Here's how the part is built. I have some questions about the finished solid (model axes, mm). Coordinates: 2 decimals unless noted, no trailing zeros. Answer in a Markdown table with one row per item. Add a question column.
Item 1: If I drill on probe 1 along Z at (x, y) = (-3, -392); probe 2 along X at (y, z) = (399, -3.5); probe 3 along X at (y, z) = (5.5, 25.5), over which ranges is the centre line in solid material (lowest first)? Write a range as from..to.
Item 2: Imagine slicing it at A-A (y = -155). State how many separate pieces and enclosed holes the cut face has, plus the area to 3 significant figures.
Item 3: I'm going to push flat-ended pins straight in: pin 1 (4.5 mm diameter, centred on x = 0, y = 75.5, fed in from -Z); pin 2 (1.2 mm diameter, centred on y = 305.5, z = -33.5, fed in from +X); pin 3 (3 mm diameter, centred on y = 133, z = 10, fed in from -X). Where does each tip first touch, or does it pass through?
from build123d import *

# Parameters (mm, degrees)
F0_R     = 2.1
F1_DEPTH = 750


with BuildPart() as f1:
    # F0 (on Front) → F1 (new body, symmetric)
    with BuildSketch(Plane.XZ):
        Polygon((-4.58, 40), (-10, 40), (-10, 34.58), (-8.2, 33.125), (-8.2, 35.5), (-6.56066, 35.5), (-3.9, 32.83934), (-3.9, 27.16066), (-6.56066, 24.5), (-8.2, 24.5), (-8.2, 26.875), (-10, 25.42), (-10, 14.58), (-8.2, 13.125), (-8.2, 15.5), (-6.56066, 15.5), (-3.9, 12.83934), (-3.9, 7.16066), (-6.56066, 4.5), (-8.2, 4.5), (-8.2, 6.875), (-10, 5.42), (-10, -5.42), (-8.2, -6.875), (-8.2, -4.5), (-6.56066, -4.5), (-3.9, -7.16066), (-3.9, -12.83934), (-6.56066, -15.5), (-8.2, -15.5), (-8.2, -13.125), (-10, -14.58), (-10, -25.42), (-8.2, -26.875), (-8.2, -24.5), (-6.56066, -24.5), (-3.9, -27.16066), (-3.9, -32.83934), (-6.56066, -35.5), (-8.2, -35.5), (-8.2, -33.125), (-10, -34.58), (-10, -40), (-4.58, -40), (-3.125, -38.2), (-5.5, -38.2), (-5.5, -36.56066), (-2.83934, -33.9), (2.83934, -33.9), (5.5, -36.56066), (5.5, -38.2), (3.125, -38.2), (4.58, -40), (10, -40), (10, -34.58), (8.2, -33.125), (8.2, -35.5), (6.56066, -35.5), (3.9, -32.83934), (3.9, -27.16066), (6.56066, -24.5), (8.2, -24.5), (8.2, -26.875), (10, -25.42), (10, -14.58), (8.2, -13.125), (8.2, -15.5), (6.56066, -15.5), (3.9, -12.83934), (3.9, -7.16066), (6.56066, -4.5), (8.2, -4.5), (8.2, -6.875), (10, -5.42), (10, 5.42), (8.2, 6.875), (8.2, 4.5), (6.56066, 4.5), (3.9, 7.16066), (3.9, 12.83934), (6.56066, 15.5), (8.2, 15.5), (8.2, 13.125), (10, 14.58), (10, 25.42), (8.2, 26.875), (8.2, 24.5), (6.56066, 24.5), (3.9, 27.16066), (3.9, 32.83934), (6.56066, 35.5), (8.2, 35.5), (8.2, 33.125), (10, 34.58), (10, 40), (4.58, 40), (3.125, 38.2), (5.5, 38.2), (5.5, 36.56066), (2.83934, 33.9), (-2.83934, 33.9), (-5.5, 36.56066), (-5.5, 38.2), (-3.125, 38.2), align=None)
        with Locations((0, -30)):
            Circle(F0_R, mode=Mode.SUBTRACT)
        Polygon((-5.93934, -17), (-2.83934, -13.9), (2.83934, -13.9), (5.93934, -17), (8.2, -17), (8.2, -23), (5.93934, -23), (2.83934, -26.1), (-2.83934, -26.1), (-5.93934, -23), (-8.2, -23), (-8.2, -17), align=None, mode=Mode.SUBTRACT)
        with Locations((0, -10)):
            Circle(F0_R, mode=Mode.SUBTRACT)
        Polygon((-5.93934, 3), (-2.83934, 6.1), (2.83934, 6.1), (5.93934, 3), (8.2, 3), (8.2, -3), (5.93934, -3), (2.83934, -6.1), (-2.83934, -6.1), (-5.93934, -3), (-8.2, -3), (-8.2, 3), align=None, mode=Mode.SUBTRACT)
        with Locations((0, 10)):
            Circle(F0_R, mode=Mode.SUBTRACT)
        Polygon((-5.93934, 23), (-2.83934, 26.1), (2.83934, 26.1), (5.93934, 23), (8.2, 23), (8.2, 17), (5.93934, 17), (2.83934, 13.9), (-2.83934, 13.9), (-5.93934, 17), (-8.2, 17), (-8.2, 23), align=None, mode=Mode.SUBTRACT)
        with Locations((0, 30)):
            Circle(F0_R, mode=Mode.SUBTRACT)
    extrude(amount=F1_DEPTH, both=True)


solid = f1.part
Here are the results:
| question | item | result |
|---|---|---|
| 1 | probe 1 | z = -34.06..-25.94, -14.06..-5.94, 5.94..14.06, 25.94..34.06 |
| 1 | probe 2 | x = -10..-5.44, 5.44..10 |
| 1 | probe 3 | x = -9.9..-8.2, -5.56..-3.44, 3.44..5.56, 8.2..9.9 |
| 2 | separate pieces | 1 |
| 2 | enclosed holes | 7 |
| 2 | area | 545 mm2 |
| 3 | pin 1 | stops at z = -33.9 |
| 3 | pin 2 | stops at x = 9.41 |
| 3 | pin 3 | stops at x = -3.9 |
